from build123d import *

# Parameters (mm, degrees)
BOSS_EXTRUDE1_DEPTH = 10
FILLET1_R           = 2
FILLET2_R           = 1


with BuildPart() as part:
    # Sketch2 → Boss-Extrude1 (new body)
    with BuildSketch(Plane(origin=(0, 0, 0), x_dir=(1, 0, 0), z_dir=(0, 1, 0))):
        with BuildLine():
            ThreePointArc((-14.8, 0), (-12.482193398, -7.952034204), (-6.254750274, -13.413355248))
            Line((-6.254750274, -13.413355248), (-5.40951375, -11.600739674))
            ThreePointArc((-5.40951375, -11.600739674), (0, 12.8), (5.40951375, -11.600739674))
            Line((5.40951375, -11.600739674), (6.254750274, -13.413355248))
            ThreePointArc((6.254750274, -13.413355248), (12.482193398, -7.952034204), (14.8, 0))
            Line((14.8, 0), (14.8, 18.453160221))
            Line((14.8, 18.453160221), (12.6, 18.453160221))
            Line((12.6, 18.453160221), (12.6, 16))
            Line((12.6, 16), (-8.8, 16))
            ThreePointArc((-8.8, 16), (-11.6, 18.8), (-8.8, 21.6))
            Line((-8.8, 21.6), (12.6, 21.6))
            Line((12.6, 21.6), (12.6, 19.453160221))
            Line((12.6, 19.453160221), (14.8, 19.453160221))
            Line((14.8, 19.453160221), (14.8, 23.6))
            Line((14.8, 23.6), (-14.8, 23.6))
            Line((-14.8, 23.6), (-14.8, 0))
        make_face()
    extrude(amount=BOSS_EXTRUDE1_DEPTH)

    # Fillet1
    fillet1_edges = [part.edges().sort_by_distance(p)[0] for p in [
        (-14.8, 5, -23.6),
    ]]
    fillet(fillet1_edges, radius=FILLET1_R)

    # Fillet2
    fillet2_edges = [part.edges().sort_by_distance(p)[0] for p in [
        (1.9, 0, -21.6),
        (1.9, 10, -21.6),
        (-11.6, 0, -18.8),
        (-11.6, 10, -18.8),
        (1.9, 0, -16),
        (1.9, 10, -16),
        (14.8, 5, -19.453160221),
        (14.8, 5, -18.453160221),
        (5.40951375, 5, 11.600739674),
        (6.254750274, 5, 13.413355248),
        (-6.254750274, 5, 13.413355248),
        (-5.40951375, 5, 11.600739674),
    ]]
    fillet(fillet2_edges, radius=FILLET2_R - 0.0001)  # a hair under: the kernel refuses the full size


solid = part.part
For this review, take the finished solid that the model builds, in its own axes (mm). A direction names the side the tool comes from. Coordinates: 2 decimals unless noted, no trailing zeros. Loops run counter-clockwise (first coordinate to the right, second up) from the corner with the lowest first, then second, coordinate; pieces in that order, holes last. Notation, with made-up numbers: (55, 67) - (84, 67) arc R6 cw to (84, 77) - close; hole circle Ø6 at (-16.5, 29.25). An arc over 180 degrees is marked (long way). Use a Markdown table: item, result. Add a question column.
Item 1: Mouldability with a two-part tool opening along Z and no side actions: class faces 6 (the face through (-6.4, 5.1, 13)), 7 (the face through (-5.77, 5.07, 11.75)), 8 (the face through (14.8, 5, -22)) as pulls with the +Z half, pulls with the -Z half, needs draft (parallel to the pull), parting line crosses it, or undercut.
Item 2: For line 1 (Z direction, x = 0, y = 5.25); line 2 (Z direction, x = 9.25, y = 5.5); line 3 (Z direction, x = -9.5, y = 6.25), list the stretches that pass through material, from the lowest coordinate up.
Item 3: We need section B-B (z = -5.5). Give the boundary of the cut face in (x, y).
Item 4: Tool access review of faces 1 (the face through (-14.2, 5.07, -23.03)), 2 (the face through (6.4, 5.1, 13)), 3 (the face through (2.05, 9.715, -21.901)), 4 (the face through (14.51, 5.07, -19.75)), 5 (the face through (2, 5, -16)): name each direction out of +Z, -Z, +X, -X, +Y, -Y from which nothing blocks a thin tool from reaching the whole face with its end or side.
Item 5: We need section D-D (x = 10.5). Give the boundary of the cut face in (y, z).
Item 6: We need section A-A (x = 0). Give the boundary of the cut face in (y, z).
Item 7: Insertion check: pin 1 Ø0.6 at (x, y) = (13, 5.5) entering from +Z; pin 2 Ø5 at (x, y) = (1, 8) entering from +Z; pin 3 Ø2.5 at (x, y) = (-1, 4.5) entering from +Z. Each pin has a flat end and moves straight along its axis. Give the tip position at first contact, or say it passes through.
Results list:
| question | item | result |
|---|---|---|
| 1 | face 6 | pulls with the +Z half |
| 1 | face 7 | undercut |
| 1 | face 8 | needs draft |
| 2 | line 1 | z = -23.6 to -21.6, -16 to -12.8 |
| 2 | line 2 | z = -23.6 to -21.6, -16 to -8.85, 8.85 to 11.55 |
| 2 | line 3 | z = -23.6 to -21.51, -16.09 to -8.58, 8.58 to 11.35 |
| 3 | outline | (-14.8, 0) - (-11.56, 0) - (-11.56, 10) - (-14.8, 10) - close; (11.56, 0) - (14.8, 0) - (14.8, 10) - (11.56, 10) - close |
| 4 | face 1 | -Z, -X, +Y, -Y |
| 4 | face 2 | +Z, +Y, -Y |
| 4 | face 3 | +Y |
| 4 | face 4 | +X, +Y, -Y |
| 4 | face 5 | +Y, -Y |
| 5 | outline | (0, -23.6) - (10, -23.6) - (10, -22.6) arc R1 ccw to (9, -21.6) - (1, -21.6) arc R1 ccw to (0, -22.6) - close; (0, -15) arc R1 ccw to (1, -16) - (9, -16) arc R1 ccw to (10, -15) - (10, -7.32) - (0, -7.32) - close; (0, 7.32) - (10, 7.32) - (10, 10.43) - (0, 10.43) - close |
| 6 | outline | (0, -23.6) - (10, -23.6) - (10, -22.6) arc R1 ccw to (9, -21.6) - (1, -21.6) arc R1 ccw to (0, -22.6) - close; (0, -15) arc R1 ccw to (1, -16) - (9, -16) arc R1 ccw to (10, -15) - (10, -12.8) - (0, -12.8) - close |
| 7 | pin 1 | stops at z = 7.6 |
| 7 | pin 2 | stops at z = -12.31 |
| 7 | pin 3 | stops at z = -12.6 |
